The listing builds one solid part. Answer for the finished solid, in the listing's coordinates (mm). A direction names the side the tool comes from. Round coordinates to 2 decimals unless told otherwise and drop trailing zeros. Order: outer loops, then holes, each group sorted by start corner. A loop starts at its lowest first (then second) coordinate and runs counter-clockwise, first axis right, second up. Notation, with made-up numbers: M 37,4 L 54,4 A21 cw 54,25 Z; hole C -13,49.5 d8. An arc over 180 degrees is marked long. Write item = value, one per line. Start each with the question number.
(1) A cutting plane is placed at D-D, the plane y = 30.55. Determine the outline of the cut face in (x, z), and give its area (3 significant figures).
(2) A cutting plane is placed at A-A, the plane z = 14.5. Determine the outline of the cut face in (x, y), and give its area (3 significant figures).
(3) For a pull along Y with two mould halves and no side action, classify faces 1 (the face through (27, 29.5, 8.6)), 2 (the face through (-1, 33, 9)), 3 (the face through (0.136, 29.134, 8.619)) as released by +Y, released by -Y, zero draft, split by the parting line, or undercut.
(4) Each of these flat-tipped pins is pushed along its axis until it touches: pin 1 (6.5 mm diameter, centred on x = 6, y = 19.5, fed in from +Z); pin 2 (1.2 mm diameter, centred on y = 19, z = 2.5, fed in from -X); pin 3 (3 mm diameter, centred on y = 17.5, z = 1.5, fed in from +X). Where does it stop, or does it pass through?
(5) A cutting plane is placed at B-B, the plane x = 21. Determine the outline of the cut face in (y, z), and give its area (3 significant figures).
(6) Straight lines are drawn through the part: probe 1 along Y at (x, z) = (5, 2.9); probe 2 along Y at (x, z) = (5, 1); probe 3 along X at (y, z) = (29.75, 1). For each, find the intervals that lie inside material, in ascending order. Write a range as from..to.
(7) A cutting plane is placed at C-C, the plane x = 12.5. Determine the outline of the cut face in (y, z), and give its area (3 significant figures).
(8) Which of the six approach directions +Z, -Z, +X, -X, +Y, -Y give full straight-line access (tool end or side, diameter ignored) to faces 4 (the face through (25, 19, 2)), 5 (the face through (12.324, 26.958, 9.002)), 6 (the face through (12, 23, 0)), 7 (the face through (21, 17, 2))?
from build123d import *

# Parameters (mm, degrees)
F0_W      = 25
F0_H      = 35
F1_DEPTH  = 4
F2_R      = 1.675
F3_DEPTH  = 25
F4_W      = 25
F4_H      = 11
F5_DEPTH  = 13
F7_DEPTH  = 6
F8_R      = 8
F9_DEPTH  = 6
F2_R_2    = 3
F10_DEPTH = 2
F11_R     = 5
F12_W     = 11
F12_H     = 17
F13_DEPTH = 2
F14_W     = 11
F14_H     = 17
F15_DEPTH = 2
F16_R     = 1.45
F17_DEPTH = 25
F18_R     = 5
F20_DEPTH = 25
F21_R     = 3


with BuildPart() as f1:
    # F0 (on Top) → F1 (new body)
    with BuildSketch(Plane.XY):
        with Locations((12.5, 17.5)):
            Rectangle(F0_W, F0_H)
    extrude(amount=F1_DEPTH)

    # F2 (on face) → F3 (cut)
    with BuildSketch(Plane.XY.offset(4)):
        with BuildLine():
            ThreePointArc((3.325, 18.5605346784), (5, 16.8855346784), (6.675, 18.5605346784))
            ThreePointArc((6.675, 18.5605346784), (5, 20.2355346784), (3.325, 18.5605346784))
        make_face()
        with Locations((20, 18.5605346784)):
            Circle(F2_R)
        with Locations((20, 3.5605346784)):
            Circle(F2_R)
        with Locations((5, 3.5605346784)):
            Circle(F2_R)
    extrude(amount=-F3_DEPTH, mode=Mode.SUBTRACT)

    # F4 (on face) → F5 (join)
    with BuildSketch(Plane.XY.offset(4)):
        with Locations((12.5, 29.5)):
            Rectangle(F4_W, F4_H)
    extrude(amount=F5_DEPTH)

    # F6 (on face) → F7 (cut)
    with BuildSketch(Plane(origin=(0, 35, 0), x_dir=(-1, 0, 0), z_dir=(0, 1, 0))):
        with BuildLine():
            ThreePointArc((-18.5, 17), (-12.5, 11), (-6.5, 17))
            Line((-6.5, 17), (-18.5, 17))
        make_face()
    extrude(amount=-F7_DEPTH, mode=Mode.SUBTRACT)

    # F8 (on face) → F9 (cut)
    with BuildSketch(Plane.XZ.offset(-24)):
        with Locations((12.5, 17)):
            Circle(F8_R)
    extrude(amount=-F9_DEPTH, mode=Mode.SUBTRACT)

    # F2 (on face) → F10 (cut)
    with BuildSketch(Plane.XY.offset(4)):
        with BuildLine():
            ThreePointArc((8, 18.5605346784), (5, 21.5605346784), (2, 18.5605346784))
            ThreePointArc((2, 18.5605346784), (5, 15.5605346784), (8, 18.5605346784))
        make_face()
        with BuildLine():
            ThreePointArc((3.325, 18.5605346784), (5, 20.2355346784), (6.675, 18.5605346784))
            ThreePointArc((6.675, 18.5605346784), (5, 16.8855346784), (3.325, 18.5605346784))
        make_face(mode=Mode.SUBTRACT)
        with Locations((20, 18.5605346784)):
            Circle(F2_R_2)
        with Locations((20, 18.5605346784)):
            Circle(F2_R, mode=Mode.SUBTRACT)
        with Locations((20, 3.5605346784)):
            Circle(F2_R_2)
        with Locations((20, 3.5605346784)):
            Circle(F2_R, mode=Mode.SUBTRACT)
        with Locations((5, 3.5605346784)):
            Circle(F2_R_2)
        with Locations((5, 3.5605346784)):
            Circle(F2_R, mode=Mode.SUBTRACT)
    extrude(amount=-F10_DEPTH, mode=Mode.SUBTRACT)

    # F11
    f11_edges = [f1.edges().sort_by_distance(p)[0] for p in [
        (0, 0, 2),
        (25, 0, 2),
    ]]
    fillet(f11_edges, radius=F11_R)

    # F12 (on face) → F13 (join)
    with BuildSketch(Plane(origin=(0, 0, 0), x_dir=(0, -1, 0), z_dir=(-1, 0, 0))):
        with Locations((-29.5, 8.5)):
            Rectangle(F12_W, F12_H)
    extrude(amount=F13_DEPTH)

    # F14 (on face) → F15 (join)
    with BuildSketch(Plane.YZ.offset(25)):
        with Locations((29.5, 8.5)):
            Rectangle(F14_W, F14_H)
    extrude(amount=F15_DEPTH)

    # F16 (on face) → F17 (cut)
    with BuildSketch(Plane.XY.offset(17)):
        with Locations((0.45, 30.55)):
            Circle(F16_R)
        with Locations((24.55, 30.55)):
            Circle(F16_R)
    extrude(amount=-F17_DEPTH, mode=Mode.SUBTRACT)

    # F18
    f18_edges = [f1.edges().sort_by_distance(p)[0] for p in [
        (-2, 24, 8.5),
        (-2, 35, 8.5),
        (27, 35, 8.5),
        (27, 24, 8.5),
    ]]
    fillet(f18_edges, radius=F18_R)

    # F19 (on face) → F20 (cut)
    with BuildSketch(Plane.XY.offset(4)):
        Polygon((5, 11.0605346784), (0, 11.0605346784), (0, 5), (0, -4.7260266729), (29.4526517391, -4.7260266729), (29.4526517391, 11.0605346784), (25, 11.0605346784), align=None)
    extrude(amount=-F20_DEPTH, mode=Mode.SUBTRACT)

    # F21
    f21_edges = [f1.edges().sort_by_distance(p)[0] for p in [
        (0, 11.060535, 2),
        (25, 11.060535, 2),
    ]]
    fillet(f21_edges, radius=F21_R)


solid = f1.part
Reported:
q1.outline = M -1.97,0 L -1,0 L -1,17 L -1.97,17 Z; M 1.9,0 L 23.1,0 L 23.1,17 L 18.5,17 A6 cw 6.5,17 L 1.9,17 Z; M 26,0 L 26.97,0 L 26.97,17 L 26,17 Z
q1.area = 337 mm²
q2.outline = M -2,29 A5 ccw 3,24 L 4.9,24 L 4.9,30 L 7.05,30 L 7.05,35 L 3,35 A5 ccw -2,30 Z; M 17.95,30 L 20.1,30 L 20.1,24 L 22,24 A5 ccw 27,29 L 27,30 A5 ccw 22,35 L 17.95,35 Z; hole C 0.45,30.55 d2.9; hole C 24.55,30.55 d2.9
q2.area = 139 mm²
q3.face_1 = zero draft
q3.face_2 = released by +Y
q3.face_3 = undercut
q4.pin_1 = 4
q4.pin_2 = 0
q4.pin_3 = 25
q5.outline = M 11.06,0 L 17.22,0 L 17.22,2 L 15.73,2 L 15.73,4 L 11.06,4 Z; M 19.9,0 L 35,0 L 35,17 L 24,17 L 24,4 L 21.39,4 L 21.39,2 L 19.9,2 Z
q5.area = 222 mm²
q6.probe_1 = 11.06..15.56, 21.56..35
q6.probe_2 = 11.06..16.89, 20.24..35
q6.probe_3 = -2..-0.76, 1.66..23.34, 25.76..27
q7.outline = M 11.06,0 L 35,0 L 35,11 L 30,11 L 30,9 L 24,9 L 24,4 L 11.06,4 Z
q7.area = 161 mm²
q8.face_4 = +Z, -Z, +X, -Y
q8.face_5 = +Z, -Y
q8.face_6 = -Z, +X, -X, +Y, -Y
q8.face_7 = +Z
